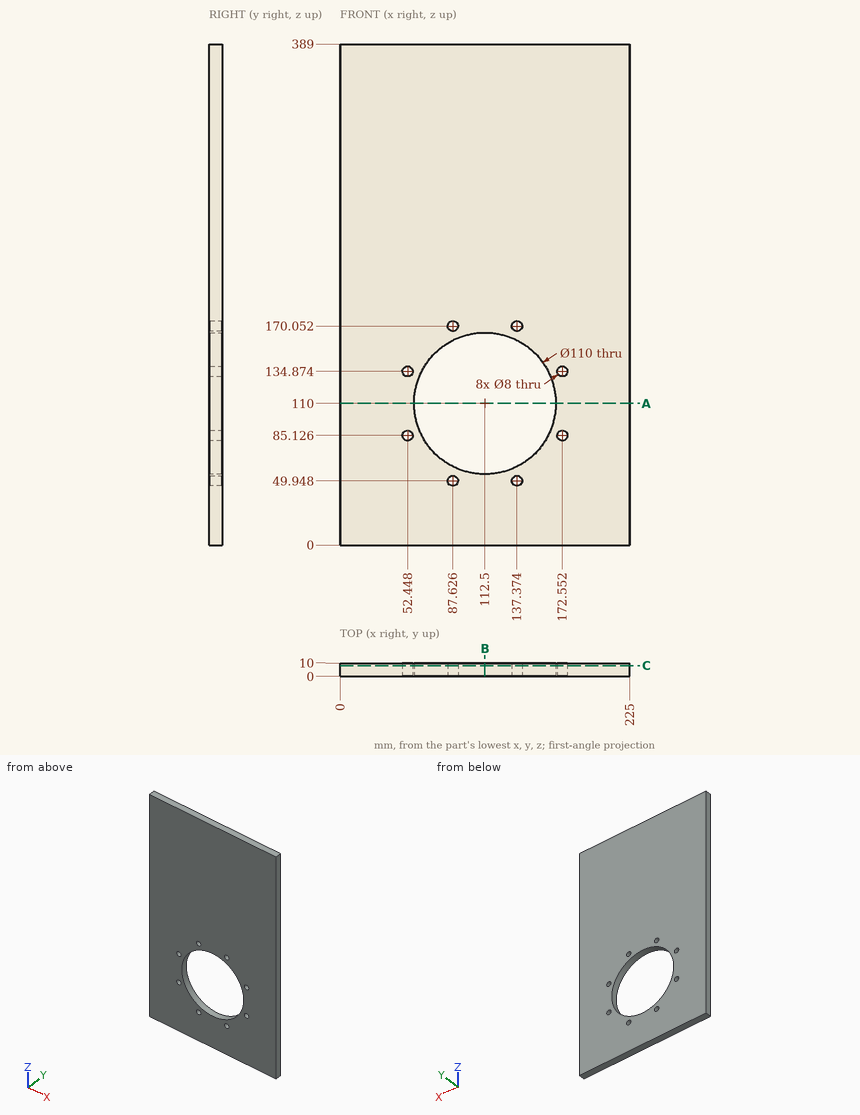
Geometry check sheet. Reference: drawing and pictorial views, mm from the part's lowest x, y, z. Coordinates: 2 decimals unless noted, no trailing zeros. Loops run counter-clockwise (first coordinate to the right, second up) from the corner with the lowest first, then second, coordinate; pieces in that order, holes last. Notation, with made-up numbers: (74.25, 67.25) -> (92.25, 67.25) arc R20 ccw to (92.25, 98.25) -> close; hole circle Ø2 at (53.25, -26.5). An arc over 180 degrees is marked (long way). Put each result on its own line as item: value.
1) Gauge pin test, flat end, axial feed: pin 1 Ø6.5 at (x, z) = (137.37, 49.95) entering from -Y. Record the tip position at first contact, or that the pin passes through.
Result set:
pin 1: passes through
2) Cross-section at A-A on z = 110. Record the boundary of the cut face in (x, y).
Result set:
outline: (0, 0) -> (57.5, 0) -> (57.5, 10) -> (0, 10) -> close; (167.5, 0) -> (225, 0) -> (225, 10) -> (167.5, 10) -> close
3) Cross-section at B-B on x = 112.5. Record the boundary of the cut face in (y, z), plus the area to 3 significant figures.
Result set:
outline: (0, 0) -> (10, 0) -> (10, 55) -> (0, 55) -> close; (0, 165) -> (10, 165) -> (10, 389) -> (0, 389) -> close
area: 2,790 mm^2
4) Cross-section at C-C on y = 8. Count the separate pieces of the cut face and the enclosed holes in it, plus the area to 3 significant figures.
Result set:
separate pieces: 1
enclosed holes: 9
area: 77,600 mm^2
5) Thickness scan on line 1 (X direction, y = 3.75, z = 111); line 2 (Z direction, x = 84, y = 3.5) (1 decimal); line 3 (Z direction, x = 148, y = 2.25). Record the ranges inside material, lowest first.
Result set:
line 1: x = 0 to 57.51, 167.49 to 225
line 2: z = 0 to 48.3, 51.6 to 63, 157 to 168.4, 171.7 to 389
line 3: z = 0 to 67.99, 152.01 to 389
